from build123d import *

# Parameters (mm, degrees)
F1_DEPTH = 250
F4_DEPTH = 10
F6_DEPTH = 108


with BuildPart() as f1:
    # F0 (on Front) → F1 (new body)
    with BuildSketch(Plane.XZ):
        with BuildLine():
            Line((-40, 25), (-40, -25))
            Line((-40, -25), (-35, -25))
            Line((-35, -25), (-35, -15))
            ThreePointArc((-35, -15), (-32.0710678119, -7.9289321881), (-25, -5))
            Line((-25, -5), (40, -5))
            Line((40, -5), (40, 25))
            Line((40, 25), (-40, 25))
        make_face()
    extrude(amount=F1_DEPTH)

    # F3 (on offset) → F4 (cut)
    with BuildSketch(Plane.XY.offset(25)):
        with BuildLine():
            Line((-14.2098601364, -131.9552626835), (29.9929159209, -131.9999964154))
            ThreePointArc((29.9929159209, -131.9999964154), (36.9999994254, -125.0028362987), (29.9985885173, -118.0000001423))
            ThreePointArc((29.9985885173, -118.0000001423), (29.9955916852, -118.0000013881), (29.992594854, -118.0000039169))
            Line((29.992594854, -118.0000039169), (-14.1923724524, -118.0467462477))
            Line((-14.1923724524, -118.0467462477), (-15.82233712, -118.0484705524))
            ThreePointArc((-15.82233712, -118.0484705524), (-21.9534147014, -125.8062406526), (-14.2098601364, -131.9552626835))
        make_face()
        with BuildLine():
            Line((-13.3595939823, -221.8050766415), (29.9685203418, -221.9999292162))
            ThreePointArc((29.9685203418, -221.9999292162), (29.9807181236, -221.9999734435), (29.9929159639, -221.9999964155))
            ThreePointArc((29.9929159639, -221.9999964155), (36.9921369062, -215.3316948665), (30.6555919845, -208.0307676786))
            Line((30.6555919845, -208.0307676786), (29.3444080155, -208.0307676786))
            Line((29.3444080155, -208.0307676786), (-14.3444080155, -208.0307676786))
            ThreePointArc((-14.3444080155, -208.0307676786), (-21.9821772076, -215.4992008031), (-13.3595939823, -221.8050766415))
        make_face()
        with BuildLine():
            Line((-14.6451076001, -41.9909978819), (29.9985885167, -41.9999998577))
            ThreePointArc((29.9985885167, -41.9999998577), (36.9999999657, -35.0006925131), (29.9999735429, -28))
            Line((29.9999735429, -28), (-14.9512298512, -28.0001698969))
            Line((-14.9512298512, -28.0001698969), (-15.0488230617, -28.0001702657))
            ThreePointArc((-15.0488230617, -28.0001702657), (-21.9970875338, -35.2019060274), (-14.6451076001, -41.9909978819))
        make_face()
    extrude(amount=-F4_DEPTH, mode=Mode.SUBTRACT)

    # F5 (on offset) → F6 (cut)
    with BuildSketch(Plane.XY.offset(25)):
        with BuildLine():
            Line((-14.9462072807, -218.9996382766), (29.9999678083, -218.9999999999))
            ThreePointArc((29.9999678083, -218.9999999999), (33.989222508, -214.7065655416), (29.4146804818, -211.0430566012))
            Line((29.4146804818, -211.0430566012), (-14.4146804818, -211.0430566012))
            ThreePointArc((-14.4146804818, -211.0430566012), (-18.9911043713, -214.7333806128), (-14.9462072807, -218.9996382766))
        make_face()
        with BuildLine():
            Line((-14.8239530385, -128.9961240555), (29.8239530385, -128.9961240555))
            Line((29.8239530385, -128.9961240555), (30.1760469615, -128.9961240555))
            ThreePointArc((30.1760469615, -128.9961240555), (33.9805586423, -125.3938945231), (30.9558331647, -121.1158806711))
            Line((30.9558331647, -121.1158806711), (29.0441668353, -121.1158806711))
            Line((29.0441668353, -121.1158806711), (-14.0441668353, -121.1158806711))
            ThreePointArc((-14.0441668353, -121.1158806711), (-18.9805586423, -124.6061054769), (-14.8239530385, -128.9961240555))
        make_face()
        with BuildLine():
            Line((-14.342635605, -38.9456142807), (29.9950937795, -38.9999969911))
            ThreePointArc((29.9950937795, -38.9999969911), (33.9999993449, -35.0022892167), (29.999672212, -31.0000000134))
            Line((29.999672212, -31.0000000134), (-14.8286087531, -31.0036735568))
            ThreePointArc((-14.8286087531, -31.0036735568), (-18.9778854783, -34.5799677135), (-15.6670414367, -38.9439898227))
            Line((-15.6670414367, -38.9439898227), (-14.342635605, -38.9456142807))
        make_face()
    extrude(amount=-F6_DEPTH, mode=Mode.SUBTRACT)


solid = f1.part
Source: CAD feature listing. Evaluate the final solid. Frame: model axes, mm. A direction names the side the tool comes from. Round coordinates to 2 decimals unless told otherwise and drop trailing zeros. Write each loop counter-clockwise with the first axis right and the second up, starting at its lowest first coordinate (ties: lowest second). Pieces come first, ordered by that corner, then holes. Notation, with made-up numbers: M 2.25,-35.5 L 31.25,-35.5 A26 ccw 31.25,-13.5 Z; hole C 40,29.25 d1. An arc over 180 degrees is marked long. One line per item, written item: value. Start each with the question number.
Item 1: Section query D-D (y = -72). Return the cut outline in (x, z), plus the area to 3 significant figures.
Item 2: Section query C-C (z = 9.5). Return the cut outline in (x, y), plus the area to 3 significant figures.
Item 3: Section query A-A (y = -215). Return the cut outline in (x, z).
Item 4: Ray query, L1, parallel to Y at x = -15, z = 17; L2, parallel to Y at x = -15, z = 5.25; L3, parallel to X at y = -215, z = 2. Return the intervals inside material, ascending. Write a range as from..to.
Item 5: Section query B-B (x = 25.5). Return the cut outline in (y, z).
Item 6: Mould query, pull axis Y, two halves, no side actions, for faces 1 (the cylindrical face through (-22, -215, 20)), 2 (the flat face through (-1, -250, 11)), 3 (the flat face through (7, -130, 15)), 4 (the flat face through (-38, -123, -25)). Classes: pulls with the +Y half, pulls with the -Y half, needs draft (parallel to the pull), parting line crosses it, or undercut.
Item 7: Set-up query: faces 5 (the flat face through (40, -123, 10)), 6 (the cylindrical face through (34, -35, 5)), 7 (the flat face through (-35, -123, -20)), 8 (the flat face through (7, -40, 15)), 9 (the flat face through (1, -151, 25)). Return all of +Z, -Z, +X, -X, +Y, -Y with unobstructed straight access to the full face (end or side cutting, diameter ignored); none if empty.
Item 8: Pin query (flat end, axial travel): pin 1 (5 mm diameter, centred on x = 11, z = 19.5, fed in from +Y); pin 2 (8 mm diameter, centred on x = 9, y = -166.5, fed in from -Z); pin 3 (12 mm diameter, centred on x = 10.5, z = -14, fed in from -Y); pin 4 (4 mm diameter, centred on x = 11, y = -122.5, fed in from +Z). Return the tip coordinate at first contact, or that it passes through.
Result set:
1. outline: M -40,-25 L -35,-25 L -35,-15 A10 cw -25,-5 L 40,-5 L 40,25 L -40,25 Z
1. area: 2,520 mm²
2. outline: M -40,-250 L 40,-250 L 40,0 L -40,0 Z; hole M -15.67,-38.94 L 30,-39 A4 ccw 30,-31 L -14.83,-31 A4 ccw Z; hole M -14.95,-219 L 30,-219 A4 ccw long 29.41,-211.04 L -14.41,-211.04 A4 ccw long Z; hole M -14.82,-129 L 30.18,-129 A4 ccw 30.96,-121.12 L -14.04,-121.12 A4 ccw long Z
2. area: 18,800 mm²
3. outline: M -40,-25 L -35,-25 L -35,-15 A10 cw -25,-5 L -19,-5 L -19,15 L -22,15 L -22,25 L -40,25 Z; M 34,-5 L 40,-5 L 40,25 L 37,25 L 37,15 L 34,15 Z
4. L1: y = -250..-222, -208..-132, -118.05..-42, -28..0
4. L2: y = -250..-219, -211..-129, -121..-38.94, -31..0
4. L3: x = -40..-19, 34..40
5. outline: M -250,-5 L -219,-5 L -219,15 L -221.98,15 L -221.98,25 L -250,25 Z; M -211.04,-5 L -129,-5 L -129,15 L -132,15 L -132,25 L -208.03,25 L -208.03,15 L -211.04,15 Z; M -121.12,-5 L -38.99,-5 L -38.99,15 L -42,15 L -42,25 L -118,25 L -118,15 L -121.12,15 Z; M -31,-5 L 0,-5 L 0,25 L -28,25 L -28,15 L -31,15 Z
6. face 1: undercut
6. face 2: pulls with the -Y half
6. face 3: undercut
6. face 4: needs draft
7. face 5: +Z, -Z, +X, +Y, -Y
7. face 6: +Z, -Z
7. face 7: -Z, +X, +Y, -Y
7. face 8: +Z
7. face 9: +Z, +X, -X, +Y, -Y
8. pin 1: stops at y = 0
8. pin 2: stops at z = -5
8. pin 3: passes through
8. pin 4: stops at z = 15
